Design review of the part built by this model. Coordinates are the model's own, in mm. Face numbers are marked on the shaded views. A direction names the side the tool comes from. Coordinates: 2 decimals unless noted, no trailing zeros. Loops run counter-clockwise (first coordinate to the right, second up) from the corner with the lowest first, then second, coordinate; pieces in that order, holes last.
Q1. Add section D-D on z = -3. Give the boundary of the cut face in (x, y).
Q2. Wall thickness on probe 1 along Y at (x, z) = (0.7, -10); probe 2 along X at (y, z) = (38, -2); probe 3 along X at (y, z) = (12, -22): over which ranges is each line inside the solid? List them lowest first.
Q3. For P1, Ø2, axis at x = 3.5, y = 23.5, coming from the -Z side; P2, Ø6, axis at x = 6, y = 10.5, coming from the -Z side; P3, Ø3, axis at x = 11, y = 7.5, coming from the -Z side; P4, Ø4, axis at y = 35, z = -10, coming from the +X side, all flat-tipped, find the tip position at first contact; note any pin that passes through.
Q4. Add section C-C on y = 21. Give the boundary of the cut face in (x, z), and give its area (3 significant figures).
Q5. Add section A-A on z = -10. Give the boundary of the cut face in (x, y), and give its area (3 significant figures).
Q6. Machinability: for the marked faces 1 and 2, which of the approach directions +Z, -Z, +X, -X, +Y, -Y give a long, thin tool a straight path to every point of the face, cutting with its end or side? Answer none if there is none.
Q7. Add section B-B on y = 5. Give the boundary of the cut face in (x, z), and give its area (3 significant figures).
```python
from build123d import *

# Parameters (mm, degrees)
EXTRUSION1_DEPTH = 40
EXTRUSION2_REACH = 17.556
ESQUISSE3_R      = 2.5
EXTRUSION3_REACH = 27.142
ESQUISSE4_R      = 1.5


with BuildPart() as part:
    # Esquisse1 → Extrusion1 (new body)
    with BuildSketch(Plane(origin=(0, 0, 0), x_dir=(1, 0, 0), z_dir=(0, 1, 0))):
        Polygon((0, 0), (0, 20), (14.142135624, 34.142135624), (15.556349186, 32.727922061), (2, 19.171572875), (2, 0), align=None)
    extrude(amount=EXTRUSION1_DEPTH)

    # Esquisse3 → Extrusion2 (cut, up to next)
    with BuildSketch(Plane.ZY, mode=Mode.PRIVATE) as extrusion2_sk1:
        with Locations((-10, 5)):
            Circle(ESQUISSE3_R)
    extrusion2_tool1 = extrude(extrusion2_sk1.sketch, amount=-EXTRUSION2_REACH, mode=Mode.PRIVATE) & part.part
    add(extrusion2_tool1.solids().sort_by_distance((0, 5, -10))[0], mode=Mode.SUBTRACT)
    # Esquisse3 → Extrusion2 (cut, up to next)
    with BuildSketch(Plane.ZY, mode=Mode.PRIVATE) as extrusion2_sk2:
        with Locations((-10, 35)):
            Circle(ESQUISSE3_R)
    extrusion2_tool2 = extrude(extrusion2_sk2.sketch, amount=-EXTRUSION2_REACH, mode=Mode.PRIVATE) & part.part
    add(extrusion2_tool2.solids().sort_by_distance((0, 35, -10))[0], mode=Mode.SUBTRACT)

    # Esquisse4 → Extrusion3 (cut, up to next)
    with BuildSketch(Plane(origin=(-10, 0, -10), x_dir=(-0.707106781, 0, 0.707106781), z_dir=(-0.707106781, 0, -0.707106781)), mode=Mode.PRIVATE) as extrusion3_sk1:
        with Locations((-24.142135624, 36)):
            Circle(ESQUISSE4_R)
    extrusion3_tool1 = extrude(extrusion3_sk1.sketch, amount=-EXTRUSION3_REACH, mode=Mode.PRIVATE) & part.part
    add(extrusion3_tool1.solids().sort_by_distance((7.071068, 36, -27.071068))[0], mode=Mode.SUBTRACT)
    # Esquisse4 → Extrusion3 (cut, up to next)
    with BuildSketch(Plane(origin=(-10, 0, -10), x_dir=(-0.707106781, 0, 0.707106781), z_dir=(-0.707106781, 0, -0.707106781)), mode=Mode.PRIVATE) as extrusion3_sk2:
        with Locations((-24.142135624, 4)):
            Circle(ESQUISSE4_R)
    extrusion3_tool2 = extrude(extrusion3_sk2.sketch, amount=-EXTRUSION3_REACH, mode=Mode.PRIVATE) & part.part
    add(extrusion3_tool2.solids().sort_by_distance((7.071068, 4, -27.071068))[0], mode=Mode.SUBTRACT)


solid = part.part
```
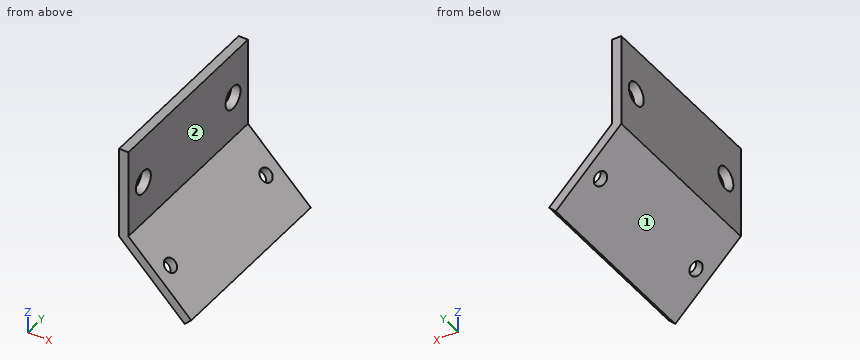
Entries:
1. outline: (0, 0) - (2, 0) - (2, 40) - (0, 40) - close
2. probe 1: y = 0 to 2.5, 7.5 to 32.5, 37.5 to 40
2. probe 2: x = 0 to 2
2. probe 3: x = 2 to 4.83
3. P1: stops at z = -24.5
3. P2: stops at z = -29
3. P3: stops at z = -32.5
3. P4: passes through
4. outline: (0, -20) - (14.14, -34.14) - (15.56, -32.73) - (2, -19.17) - (2, 0) - (0, 0) - close
4. area: 78.3 mm2
5. outline: (0, 0) - (2, 0) - (2, 2.5) - (0, 2.5) - close; (0, 7.5) - (2, 7.5) - (2, 32.5) - (0, 32.5) - close; (0, 37.5) - (2, 37.5) - (2, 40) - (0, 40) - close
5. area: 60.0 mm2
6. face 1: -Z, -X, +Y, -Y
6. face 2: +Z, +X, +Y, -Y
7. outline: (0, -20) - (6.28, -26.28) - (7.69, -24.87) - (2, -19.17) - (2, -12.5) - (0, -12.5) - close; (0, -7.5) - (2, -7.5) - (2, 0) - (0, 0) - close; (7.86, -27.86) - (14.14, -34.14) - (15.56, -32.73) - (9.28, -26.45) - close
7. area: 63.9 mm2
